```python
from build123d import *

# Parameters (mm, degrees)
BOSS_EXTRUDE1_DEPTH = 3.175
CUT_EXTRUDE1_DEPTH  = 4.175


with BuildPart() as part:
    # Sketch1 → Boss-Extrude1 (new body)
    with BuildSketch(Plane.XY):
        Polygon((-33.3375, 149.225), (-58.7375, 149.225), (-58.7375, 146.05), (-74.6125, 146.05), (-74.6125, 127), (-77.7875, 127), (-77.7875, 101.6), (-74.6125, 101.6), (-74.6125, 85.725), (-77.7875, 85.725), (-77.7875, 60.325), (-74.6125, 60.325), (-74.6125, 41.275), (-77.7875, 41.275), (-77.7875, 15.875), (-74.6125, 15.875), (-74.6125, 0), (-55.5625, 0), (-55.5625, -3.175), (-30.1625, -3.175), (-30.1625, 0), (-14.2875, 0), (-14.2875, -3.175), (11.1125, -3.175), (11.1125, 0), (30.1625, 0), (30.1625, -3.175), (55.5625, -3.175), (55.5625, 0), (71.4375, 0), (71.4375, 19.05), (74.6125, 19.05), (74.6125, 44.45), (71.4375, 44.45), (71.4375, 60.325), (74.6125, 60.325), (74.6125, 85.725), (71.4375, 85.725), (71.4375, 104.775), (74.6125, 104.775), (74.6125, 130.175), (71.4375, 130.175), (71.4375, 146.05), (52.3875, 146.05), (52.3875, 149.225), (26.9875, 149.225), (26.9875, 146.05), (11.1125, 146.05), (11.1125, 149.225), (-14.2875, 149.225), (-14.2875, 146.05), (-33.3375, 146.05), align=None)
    extrude(amount=BOSS_EXTRUDE1_DEPTH)

    # Sketch2 → Cut-Extrude1 (cut, through all)
    with BuildSketch(Plane.XY.offset(3.175)):
        Polygon((-38.1, 73.025), (0, 73.025), (0, 111.125), (-15.781536726, 111.125), (-38.1, 88.806536726), align=None)
        Polygon((0, 111.125), (0, 73.025), (38.1, 73.025), (38.1, 88.806536726), (15.781536726, 111.125), align=None)
        Polygon((0, 73.025), (0, 34.925), (15.781536726, 34.925), (38.1, 57.243463274), (38.1, 73.025), align=None)
        Polygon((-15.781536726, 34.925), (0, 34.925), (0, 73.025), (-38.1, 73.025), (-38.1, 57.243463274), align=None)
    extrude(amount=-CUT_EXTRUDE1_DEPTH, mode=Mode.SUBTRACT)


solid = part.part
```
Source: CAD feature listing. Evaluate the final solid. Frame: model axes, mm. A direction names the side the tool comes from. Round coordinates to 2 decimals unless told otherwise and drop trailing zeros. Loops run counter-clockwise (first coordinate to the right, second up) from the corner with the lowest first, then second, coordinate; pieces in that order, holes last.
1. Mould query, pull axis X, two halves, no side actions, for faces 1 (the flat face through (-27.097, 46.24, 1.61)), 2 (the flat face through (-37, 91, 0)). Classes: released by +X, released by -X, zero draft, split by the parting line, or undercut.
2. Section query A-A on x = 8. Output: boundary loops of the cut face in (y, z) (3 decimals).
3. Access query for faces 3 (the flat face through (-37, 91, 3.175)), 4 (the flat face through (27.097, 99.81, 1.61)). Directions: +Z, -Z, +X, -X, +Y, -Y. A direction counts if a zero-diameter tool reaches every point of the face in a straight line with its end or side. Return the directions, or none.
4. Section query B-B on y = 82. Output: boundary loops of the cut face in (x, z) (1 decimal), and give its area (3 significant figures).
5. Section query C-C on y = 136. Output: boundary loops of the cut face in (x, z) (1 decimal), and give its area (3 significant figures).
6. Section query D-D on x = 64. Output: boundary loops of the cut face in (y, z) (3 decimals).
7. Contact query for flat-ended pins moving along their axis: pin 1 (1 mm diameter, centred on y = 147.5, z = 1.5, fed in from +X); pin 2 (1.6 mm diameter, centred on x = -65, z = 2, fed in from +Y); pin 3 (1 mm diameter, centred on x = -76, z = 2, fed in from +Y). Output: stop coordinate, or through.
8. Ray query, L1, parallel to Y at x = 8, z = 1.5 (3 decimals); L2, parallel to X at y = 73, z = 1.1; L3, parallel to Y at x = -71.5, z = 2.4. Return the intervals inside material, ascending.
Answers below:
1. face 1: undercut
1. face 2: zero draft
2. outline: (-3.175, 0) - (34.925, 0) - (34.925, 3.175) - (-3.175, 3.175) - close; (111.125, 0) - (149.225, 0) - (149.225, 3.175) - (111.125, 3.175) - close
3. face 3: +Z, +X, -X, +Y, -Y
3. face 4: +Z, -Z
4. outline: (-77.8, 0) - (-38.1, 0) - (-38.1, 3.2) - (-77.8, 3.2) - close; (38.1, 0) - (74.6, 0) - (74.6, 3.2) - (38.1, 3.2) - close
4. area: 242 mm2
5. outline: (-74.6, 0) - (71.4, 0) - (71.4, 3.2) - (-74.6, 3.2) - close
5. area: 464 mm2
6. outline: (0, 0) - (146.05, 0) - (146.05, 3.175) - (0, 3.175) - close
7. pin 1: stops at x = 52.39
7. pin 2: stops at y = 146.05
7. pin 3: stops at y = 127
8. L1: y = -3.175 to 34.925, 111.125 to 149.225
8. L2: x = -77.79 to -38.1, 38.1 to 74.61
8. L3: y = 0 to 146.05
